Verification items for this drawing (mm, ordinates from the low corner). Round coordinates to 2 decimals unless told otherwise and drop trailing zeros. Order: outer loops, then holes, each group sorted by start corner. A loop starts at its lowest first (then second) coordinate and runs counter-clockwise, first axis right, second up.
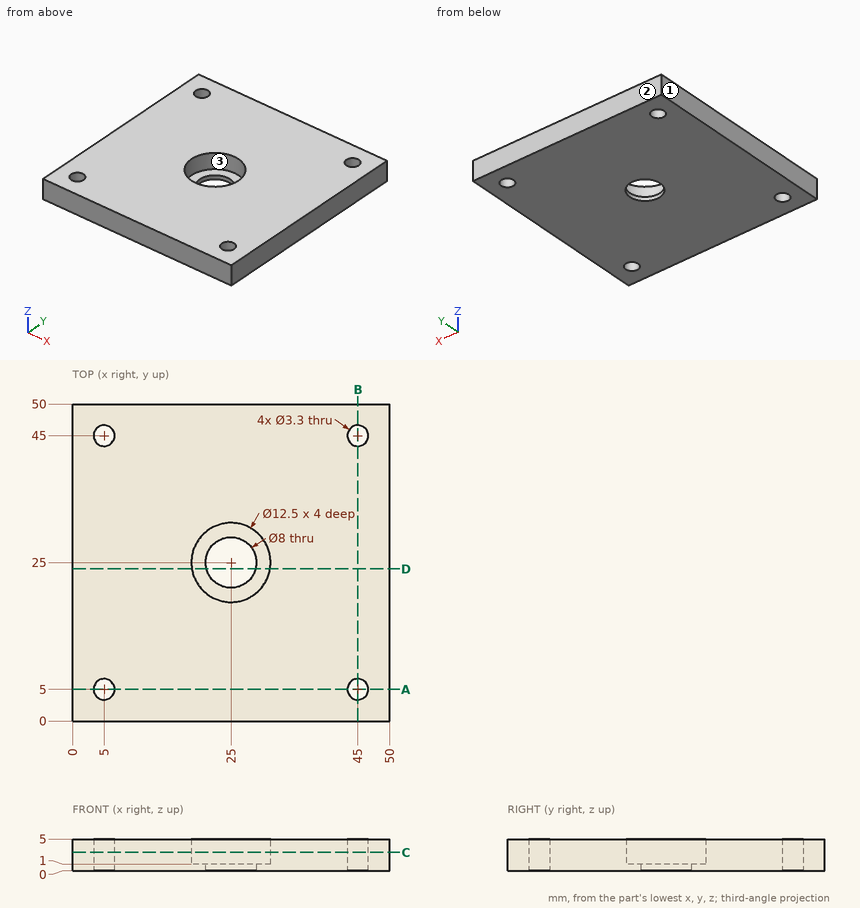
Item 1: Sectioned sample at C-C (z = 2.9). Record the cut outline in (x, y), and give its area (3 significant figures).
Answer:
outline: (0, 0) - (50, 0) - (50, 50) - (0, 50) - close; hole circle Ø3.3 at (5, 5); hole circle Ø3.3 at (5, 45); hole circle Ø12.5 at (25, 25); hole circle Ø3.3 at (45, 5); hole circle Ø3.3 at (45, 45)
area: 2,340 mm2
Item 2: Scan lines: line 1 along Y through (x, z) = (45, 1.5); line 2 along X through (y, z) = (46, 3.8); line 3 along Y through (x, z) = (25, 0.3). Record each from-to range of solid material in increasing order.
Answer:
line 1: y = 0 to 3.35, 6.65 to 43.35, 46.65 to 50
line 2: x = 0 to 3.69, 6.31 to 43.69, 46.31 to 50
line 3: y = 0 to 21, 29 to 50
Item 3: Sectioned sample at D-D (y = 24). Record the cut outline in (x, z), and give its area (3 significant figures).
Answer:
outline: (0, 0) - (21.13, 0) - (21.13, 1) - (18.83, 1) - (18.83, 5) - (0, 5) - close; (28.87, 0) - (50, 0) - (50, 5) - (31.17, 5) - (31.17, 1) - (28.87, 1) - close
area: 193 mm2
Item 4: Sectioned sample at A-A (y = 5). Record the cut outline in (x, z).
Answer:
outline: (0, 0) - (3.35, 0) - (3.35, 5) - (0, 5) - close; (6.65, 0) - (43.35, 0) - (43.35, 5) - (6.65, 5) - close; (46.65, 0) - (50, 0) - (50, 5) - (46.65, 5) - close
Item 5: Go/stop test with flat-tipped pins: P1, Ø7, axis at x = 25, y = 25, coming from the +Z side; P2, Ø10, axis at x = 25, y = 25, coming from the +Z side. Record where each tip stops, or that it passes through.
Answer:
P1: passes through
P2: stops at z = 1
Item 6: Release check for a two-part mould opening along X. For the marked faces 1, 2 and 3 record: released by +X, released by -X, zero draft, split by the parting line, or undercut.
Answer:
face 1: released by -X
face 2: zero draft
face 3: undercut
